```python
from build123d import *

# Parameters (mm, degrees)
SKETCH2_W           = 7.8
SKETCH2_H           = 17.8
BOSS_EXTRUDE1_DEPTH = 9.9
SKETCH3_W           = 3.4
SKETCH3_H           = 11.85
CUT_EXTRUDE1_DEPTH  = 9.9
SKETCH5_R           = 2.25
BOSS_EXTRUDE2_DEPTH = 3.6
BOSS_EXTRUDE3_START = 3.6
SKETCH6_R           = 2.25
BOSS_EXTRUDE3_DEPTH = 3.6


with BuildPart() as part:
    # Sketch2 → Boss-Extrude1 (new body)
    with BuildSketch(Plane.XY):
        with Locations((3.852048319, 8.842226891)):
            Rectangle(SKETCH2_W, SKETCH2_H)
    extrude(amount=BOSS_EXTRUDE1_DEPTH)

    # Sketch3 → Cut-Extrude1 (cut)
    with BuildSketch(Plane.XY.offset(9.9)):
        with Locations((3.852048319, 8.842226891)):
            Rectangle(SKETCH3_W, SKETCH3_H)
    extrude(amount=-CUT_EXTRUDE1_DEPTH, mode=Mode.SUBTRACT)

    # Sketch5 → Boss-Extrude2 (add)
    with BuildSketch(Plane(origin=(7.752048319, 0, 0), x_dir=(0, 0, -1), z_dir=(1, 0, 0))):
        with Locations(Location((-4.95, 8.842226891, 0), (0, 0, 90))):
            Circle(SKETCH5_R)
    extrude(amount=BOSS_EXTRUDE2_DEPTH)

    # Sketch6 → Boss-Extrude3 (add)
    with BuildSketch(Plane.ZY.offset(0.047951681).offset(BOSS_EXTRUDE3_START)):
        with Locations(Location((4.95, 8.842226891, 0), (0, 0, 90))):
            Circle(SKETCH6_R)
    extrude(amount=-BOSS_EXTRUDE3_DEPTH)


solid = part.part
```
Geometry check sheet. Reference: the model listing, model coordinates, mm. A direction names the side the tool comes from. Coordinates: 2 decimals unless noted, no trailing zeros. Order: outer loops, then holes, each group sorted by start corner. A loop starts at its lowest first (then second) coordinate and runs counter-clockwise, first axis right, second up.
Q1. Sectioned sample at D-D on z = 4.95. Record the cut outline in (x, y), and give its area (3 significant figures).
Reply:
outline: (-3.65, 6.59) - (-0.05, 6.59) - (-0.05, -0.06) - (7.75, -0.06) - (7.75, 6.59) - (11.35, 6.59) - (11.35, 11.09) - (7.75, 11.09) - (7.75, 17.74) - (-0.05, 17.74) - (-0.05, 11.09) - (-3.65, 11.09) - close; hole (2.15, 2.92) - (5.55, 2.92) - (5.55, 14.77) - (2.15, 14.77) - close
area: 131 mm2
Q2. Sectioned sample at C-C on y = 8.5. Record the cut outline in (x, z).
Reply:
outline: (-3.65, 2.73) - (-0.05, 2.73) - (-0.05, 0) - (2.15, 0) - (2.15, 9.9) - (-0.05, 9.9) - (-0.05, 7.17) - (-3.65, 7.17) - close; (5.55, 0) - (7.75, 0) - (7.75, 2.73) - (11.35, 2.73) - (11.35, 7.17) - (7.75, 7.17) - (7.75, 9.9) - (5.55, 9.9) - close
Q3. Draft check along Y on faces 1 (the face through (11.352, 9, 5)), 2 (the face through (2.152, 9, 5)), 3 (the face through (-1.873, 7.057, 6.319)). Enter one of: released by +Y, released by -Y, zero draft, split by the parting line, or undercut.
Reply:
face 1: zero draft
face 2: undercut
face 3: split by the parting line
Q4. Sectioned sample at A-A on y = 12.25. Record the cut outline in (x, z).
Reply:
outline: (-0.05, 0) - (2.15, 0) - (2.15, 9.9) - (-0.05, 9.9) - close; (5.55, 0) - (7.75, 0) - (7.75, 9.9) - (5.55, 9.9) - close
Q5. Thickness scan on probe 1 along X at (y, z) = (6.25, 6.75); probe 2 along X at (y, z) = (8.5, 4); probe 3 along Y at (x, z) = (3.25, 4). Record the ranges inside material, lowest first.
Reply:
probe 1: x = -0.05 to 2.15, 5.55 to 7.75
probe 2: x = -3.65 to 2.15, 5.55 to 11.35
probe 3: y = -0.06 to 2.92, 14.77 to 17.74
Q6. Depth check by flat-ended pin: pin 1 Ø4 at (y, z) = (3, 4.5) entering from +X; pin 2 Ø1.5 at (y, z) = (13, 9) entering from -X. Enter the tip coordinate at first touch or a pass-through.
Reply:
pin 1: stops at x = 7.75
pin 2: stops at x = -0.05
Q7. Sectioned sample at B-B on z = 1.5. Record the cut outline in (x, y), and give its area (4 significant figures).
Reply:
outline: (-0.05, -0.06) - (7.75, -0.06) - (7.75, 17.74) - (-0.05, 17.74) - close; hole (2.15, 2.92) - (5.55, 2.92) - (5.55, 14.77) - (2.15, 14.77) - close
area: 98.55 mm2
Q8. Tool access check on faces 4 (the face through (2, 9, 9.9)), 5 (the face through (-0.048, 6.7, 3.8)), 6 (the face through (-3.648, 9, 5)), 7 (the face through (7.752, 6.7, 3.8)), 8 (the face through (4, 2.917, 5)). Record the directions out of +Z, -Z, +X, -X, +Y, -Y that give a thin tool (end or side, any length) a straight path to the whole face; none if there is none.
Reply:
face 4: +Z, +X, -X, +Y, -Y
face 5: -X
face 6: +Z, -Z, -X, +Y, -Y
face 7: +X
face 8: +Z, -Z
